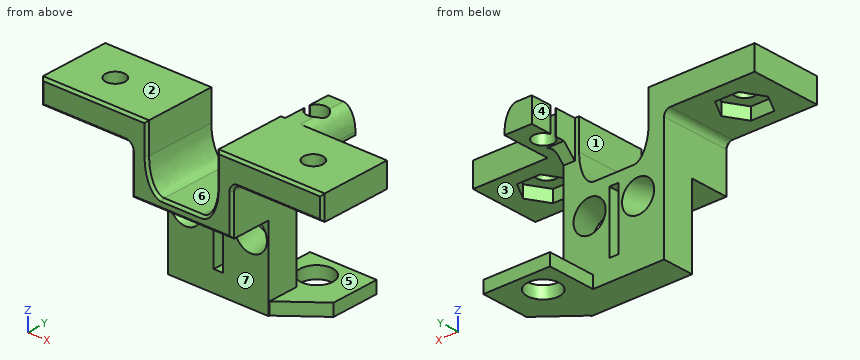
```python
from build123d import *

# Parameters (mm, degrees)
BOSS_EXTRUDE1_DEPTH = 12
CUT_EXTRUDE1_DEPTH  = 2
SKETCH3_W           = 16.6
SKETCH3_H           = 13.4
BOSS_EXTRUDE2_DEPTH = 5.2
SKETCH5_R           = 1.6
CUT_EXTRUDE2_DEPTH  = 5
SKETCH6_W           = 4.5
SKETCH6_H           = 4
BOSS_EXTRUDE4_DEPTH = 8
CUT_EXTRUDE4_DEPTH  = 7
SKETCH8_R           = 2.65
CUT_EXTRUDE5_DEPTH  = 7
SKETCH10_R          = 2.65
CUT_EXTRUDE6_DEPTH  = 7
CHAMFER2_SIZE       = 2
SKETCH12_W          = 3
SKETCH12_H          = 2
SKETCH12_W_2        = 6.148694825
SKETCH12_W_3        = 1.851305175
BOSS_EXTRUDE5_DEPTH = 8
SKETCH13_R          = 2.65
CUT_EXTRUDE7_DEPTH  = 3
CHAMFER4_SIZE       = 5
CHAMFER4_SIZE_2     = 6.174485783
SKETCH16_W          = 1.5
SKETCH16_H          = 10
CUT_EXTRUDE8_DEPTH  = 11
CHAMFER5_SIZE       = 0.4
FILLET1_SIZE        = 2
FILLET1_SIZE_2      = 3.5


with BuildPart() as part:
    # Sketch1 → Boss-Extrude1 (new body)
    with BuildSketch(Plane(origin=(0, 0, 0), x_dir=(1, 0, 0), z_dir=(0, 1, 0))):
        with BuildLine():
            Line((-23.25, -5), (-5.749755012, -5))
            Line((-5.749755012, -5), (-5.749755012, 0))
            add(Edge.make_bspline(
                [(-3.25, 5), (-5.749755012, 5), (-5.749755012, 0)],
                knots=[0, 0, 0, 1.570796327, 1.570796327, 1.570796327], degree=2, weights=[1, 0.707106781, 1]))
            Line((-3.25, 5), (3.25, 5))
            add(Edge.make_bspline(
                [(5.748694825, 0), (5.748694825, 5), (3.25, 5)],
                knots=[4.71238898, 4.71238898, 4.71238898, 6.283185307, 6.283185307, 6.283185307], degree=2, weights=[1, 0.707106781, 1]))
            Line((5.748694825, 0), (5.748694825, -5))
            Line((5.748694825, -5), (23.25, -5))
            Line((23.25, -5), (23.25, -3))
            Line((23.25, -3), (23.25, -1))
            Line((23.25, -1), (9.3, -1))
            ThreePointArc((9.3, -1), (8.592893219, -0.707106781), (8.3, 0))
            Line((8.3, 0), (8.3, 6.6))
            Line((8.3, 6.6), (-8.3, 6.6))
            Line((-8.3, 6.6), (-8.3, 0))
            ThreePointArc((-8.3, 0), (-8.592893219, -0.707106781), (-9.3, -1))
            Line((-9.3, -1), (-23.25, -1))
            Line((-23.25, -1), (-23.25, -5))
        make_face()
    extrude(amount=BOSS_EXTRUDE1_DEPTH)

    # Sketch2 → Cut-Extrude1 (cut)
    with BuildSketch(Plane(origin=(0, 0, 1), x_dir=(-1, 0, 0), z_dir=(0, 0, -1))):
        Polygon((20.147177825, 6), (18.213054423, 9.35), (14.344807619, 9.35), (12.410684218, 6), (14.344807619, 2.65), (18.213054423, 2.65), align=None)
        Polygon((-12.542169585, 6), (-14.476292987, 9.35), (-18.34453979, 9.35), (-20.278663192, 6), (-18.34453979, 2.65), (-14.476292987, 2.65), align=None)
    extrude(amount=-CUT_EXTRUDE1_DEPTH, mode=Mode.SUBTRACT)

    # Sketch3 → Boss-Extrude2 (add)
    with BuildSketch(Plane(origin=(0, 12, 0), x_dir=(1, 0, 0), z_dir=(0, 1, 0))):
        with Locations((0, 13.3)):
            Rectangle(SKETCH3_W, SKETCH3_H)
    extrude(amount=-BOSS_EXTRUDE2_DEPTH)

    # Sketch5 → Cut-Extrude2 (cut)
    with BuildSketch(Plane(origin=(0, 0, 1), x_dir=(-1, 0, 0), z_dir=(0, 0, -1))):
        with Locations((-16.410416388, 6)):
            Circle(SKETCH5_R)
        with Locations((16.278931021, 6)):
            Circle(SKETCH5_R)
    extrude(amount=-CUT_EXTRUDE2_DEPTH, mode=Mode.SUBTRACT)

    # Sketch6 → Boss-Extrude4 (add)
    with BuildSketch(Plane(origin=(0, 12, 0), x_dir=(1, 0, 0), z_dir=(0, 1, 0))):
        with Locations((8.698694825, -3)):
            Rectangle(SKETCH6_W, SKETCH6_H)
    extrude(amount=BOSS_EXTRUDE4_DEPTH)

    # Sketch7 → Cut-Extrude4 (cut)
    with BuildSketch(Plane(origin=(0, 0, 1), x_dir=(-1, 0, 0), z_dir=(0, 0, -1))):
        with BuildLine():
            ThreePointArc((-6.448694825, 16), (-6.468205549, 16.252991544), (-6.526276305, 16.5))
            Line((-6.526276305, 16.5), (-7.999397269, 16.5))
            Line((-7.999397269, 16.5), (-7.999397269, 15.5))
            Line((-7.999397269, 15.5), (-6.526276305, 15.5))
            ThreePointArc((-6.526276305, 15.5), (-6.468205549, 15.747008456), (-6.448694825, 16))
        make_face()
        with BuildLine():
            Line((-7.999397269, 16.5), (-6.526276305, 16.5))
            ThreePointArc((-6.526276305, 16.5), (-9.748694825, 16), (-6.526276305, 15.5))
            Line((-6.526276305, 15.5), (-7.999397269, 15.5))
            Line((-7.999397269, 15.5), (-7.999397269, 16.5))
        make_face()
        with BuildLine():
            Line((-6.448694825, 15.5), (-6.448694825, 16))
            ThreePointArc((-6.448694825, 16), (-6.468205549, 15.747008456), (-6.526276305, 15.5))
            Line((-6.526276305, 15.5), (-6.448694825, 15.5))
        make_face()
        with BuildLine():
            Line((-6.448694825, 16), (-6.448694825, 16.5))
            Line((-6.448694825, 16.5), (-6.526276305, 16.5))
            ThreePointArc((-6.526276305, 16.5), (-6.468205549, 16.252991544), (-6.448694825, 16))
        make_face()
    extrude(amount=-CUT_EXTRUDE4_DEPTH, mode=Mode.SUBTRACT)

    # Sketch8 → Cut-Extrude5 (cut, along a direction that is not the sketch's normal)
    with BuildSketch(Plane(origin=(0, 12, 0), x_dir=(1, 0, 0), z_dir=(0, 1, 0))):
        with Locations((-4, 9.6)):
            Circle(SKETCH8_R)
    extrude(amount=-CUT_EXTRUDE5_DEPTH, dir=(0.2588190451025147, 0.96592582628907, -1.457918124587514e-13), mode=Mode.SUBTRACT)

    # Sketch10 → Cut-Extrude6 (cut, along a direction that is not the sketch's normal)
    with BuildSketch(Plane(origin=(0, 12, 0), x_dir=(1, 0, 0), z_dir=(0, 1, 0))):
        with Locations((4, 9.6)):
            Circle(SKETCH10_R)
    extrude(amount=-CUT_EXTRUDE6_DEPTH, dir=(-0.25881904510251447, 0.96592582628907, 0), mode=Mode.SUBTRACT)

    # Chamfer2
    chamfer2_edges = [part.edges().sort_by_distance(p)[0] for p in [
        (7.874347412, 12, 1),
    ]]
    chamfer(chamfer2_edges, length=CHAMFER2_SIZE)

    # Sketch12 → Boss-Extrude5 (add)
    with BuildSketch(Plane(origin=(0, 12, 0), x_dir=(1, 0, 0), z_dir=(0, 1, 0))):
        with Locations((4.948694825, 19)):
            Rectangle(SKETCH12_W, SKETCH12_H)
        with Locations((11.374347413, 19)):
            Rectangle(SKETCH12_W_2, SKETCH12_H)
        with Locations((7.374347413, 19)):
            Rectangle(SKETCH12_W_3, SKETCH12_H)
    extrude(amount=BOSS_EXTRUDE5_DEPTH)

    # Sketch13 → Cut-Extrude7 (cut)
    with BuildSketch(Plane(origin=(0, 0, -20), x_dir=(-1, 0, 0), z_dir=(0, 0, -1))):
        with Locations((-8.098694825, 16)):
            Circle(SKETCH13_R)
    extrude(amount=-CUT_EXTRUDE7_DEPTH, mode=Mode.SUBTRACT)

    # Chamfer4
    # the kernel refuses this chamfer: 6.174485783, 5 mm, written as the material it adds along each edge
    with BuildSketch(Plane(origin=(8.3, 12, -18), x_dir=(-0.037204697112204525, -0.9993076655929289, 0), z_dir=(0, 0, -1))) as chamfer4_piece_1_section:
        Polygon((CHAMFER4_SIZE * 0.999307665593, -CHAMFER4_SIZE * 0.0372046971122), (-CHAMFER4_SIZE_2 * 0.0372046971102, -CHAMFER4_SIZE_2 * 0.99930766554), (0, 0), align=None)
    chamfer4_piece_1 = extrude(amount=2, mode=Mode.PRIVATE)
    chamfer4_piece_1 = split(chamfer4_piece_1, bisect_by=Plane(origin=(14.448694825, 10.333304375, -19), z_dir=(-1, 0, 0)), keep=Keep.TOP, mode=Mode.PRIVATE)
    add(chamfer4_piece_1)

    # Sketch16 → Cut-Extrude8 (cut)
    with BuildSketch(Plane.XZ.offset(-6.8)):
        with Locations((0, -11.6)):
            Rectangle(SKETCH16_W, SKETCH16_H)
    extrude(amount=-CUT_EXTRUDE8_DEPTH, mode=Mode.SUBTRACT)

    # Chamfer5
    chamfer5_edges = [part.edges().sort_by_distance(p)[0] for p in [
        (0, 0, -5),
        (-5.260112096, 0, -2.972310439),
        (-5.749755012, 0, 2.5),
        (-14.499877506, 0, 5),
        (-23.25, 0, 3),
        (-16.275, 0, 1),
        (-8.592893219, 0, 0.707106781),
        (-8.3, 0, -3.3),
        (0, 0, -6.6),
        (8.3, 0, -3.3),
        (8.592893219, 0, 0.707106781),
        (16.275, 0, 1),
        (23.25, 0, 3),
        (14.499347412, 0, 5),
        (5.748694825, 0, 2.5),
        (5.259369228, 0, -2.972013605),
    ]]
    chamfer(chamfer5_edges, length=CHAMFER5_SIZE)

    # Fillet1
    # an asymmetric fillet: 3.5, 2 mm, written as the material it takes off along each edge
    with BuildSketch(Plane(origin=(10.948694825, 12, 5), x_dir=(-1, 0, 0), z_dir=(0, 1, 0))) as fillet1_piece_1:
        with BuildLine():
            Bezier((FILLET1_SIZE, 0), (0, 0), (0, -FILLET1_SIZE_2), weights=[1, 0.707106781, 1])
            Line((0, -FILLET1_SIZE_2), (0, 0))
            Line((0, 0), (FILLET1_SIZE, 0))
        make_face()
    extrude(amount=16.75, mode=Mode.SUBTRACT)


solid = part.part
```
Geometry: final body of the model. Coordinates: model frame, mm. Face numbers are marked on the shaded views. A direction names the side the tool comes from. Round coordinates to 2 decimals unless told otherwise and drop trailing zeros. Order: outer loops, then holes, each group sorted by start corner. A loop starts at its lowest first (then second) coordinate and runs counter-clockwise, first axis right, second up. Notation, with made-up numbers: (-8, 20.25) -> (10, 20.25) arc R26 ccw to (10, 41.25) -> close; hole circle Ø2 at (58, -7). An arc over 180 degrees is marked (long way). Use one line per item in the form item = value.
(1) Access query for the marked faces 4, 5, 6 and 7. Directions: +Z, -Z, +X, -X, +Y, -Y. A direction counts if a zero-diameter tool reaches every point of the face in a straight line with its end or side. Return the directions, or none.
Results list:
face_4 = +Z, -X, +Y
face_5 = +X, +Y
face_6 = +Z, +Y, -Y
face_7 = -Z, +X, -X, -Y
(2) First-contact query: pin 1 Ø3 at (x, y) = (0.5, 8.5) entering from +Z; pin 2 Ø10.5 at (x, z) = (1, -12) entering from -Y; pin 3 Ø4.5 at (x, z) = (15, 2.5) entering from +Y. Flat tips, straight axial feed; report the tip coordinate or a pass-through.
Results list:
pin_1 = -5
pin_2 = 6.8
pin_3 = 12
(3) Section B-B on x = 19.5. Return loops of the section in (y, z), and give its area (3 significant figures).
Results list:
outline = (0, 1.4) -> (0.4, 1) -> (4.65, 1) -> (4.65, 3) -> (7.35, 3) -> (7.35, 1) -> (12, 1) -> (12, 5) -> (0.4, 5) -> (0, 4.6) -> close
area = 42.4 mm^2
(4) Section A-A on z = -14.5. Return loops of the section in (x, y).
Results list:
outline = (-8.3, 6.8) -> (-0.75, 6.8) -> (-0.75, 12) -> (-8.3, 12) -> close; (0.75, 6.8) -> (8.3, 6.8) -> (8.3, 12) -> (0.75, 12) -> close
(5) Ray query, probe 1 along Y at (x, z) = (6, -16); probe 2 along Z at (x, y) = (-19, 6.75); probe 3 along X at (y, z) = (3, -4.75). Return the intervals inside material, ascending. Write a range as [from, to].
Results list:
probe_1 = [6.8, 12]
probe_2 = [3, 5]
probe_3 = [-8.3, -4.03], [4.03, 8.3]
(6) Draft query along Z for the marked faces 1, 2 and 3. Return one class per face: pulls with the +Z half, pulls with the -Z half, needs draft (parallel to the pull), parting line crosses it, or undercut.
Results list:
face_1 = needs draft
face_2 = pulls with the +Z half
face_3 = undercut
(7) Section C-C on z = -8.5. Count the separate pieces of the cut face and the enclosed holes in it, and give its area (3 significant figures).
Results list:
separate_pieces = 4
enclosed_holes = 0
area = 28.4 mm^2
